```python
from build123d import *

# Parameters (mm, degrees)
SKETCH1_W           = 250
SKETCH1_H           = 100
SKETCH1_R           = 5
SKETCH1_R_2         = 2.5
BOSS_EXTRUDE1_DEPTH = 5
BOSS_EXTRUDE2_DEPTH = 10
CUT_EXTRUDE1_DEPTH  = 5
SKETCH4_R           = 4
CUT_EXTRUDE2_DEPTH  = 44.5
SKETCH5_W           = 5
SKETCH5_H           = 5
SKETCH5_W_2         = 2.5
CUT_EXTRUDE3_DEPTH  = 290.5
SKETCH6_W           = 5
SKETCH6_H           = 5
CUT_EXTRUDE4_DEPTH  = 290.5


with BuildPart() as part:
    # Sketch1 → Boss-Extrude1 (new, symmetric)
    with BuildSketch(Plane(origin=(0, 0, 0), x_dir=(1, 0, 0), z_dir=(0, 1, 0))):
        Rectangle(SKETCH1_W, SKETCH1_H)
        with Locations(Location((-100, 40, 0), (0, 0, 270))):
            Circle(SKETCH1_R, mode=Mode.SUBTRACT)
        with Locations(Location((100, 40, 0), (0, 0, 270))):
            Circle(SKETCH1_R, mode=Mode.SUBTRACT)
        with Locations(Location((-100, -40, 0), (0, 0, 90))):
            Circle(SKETCH1_R, mode=Mode.SUBTRACT)
        with Locations(Location((100, -40, 0), (0, 0, 90))):
            Circle(SKETCH1_R, mode=Mode.SUBTRACT)
        with Locations(Location((-20, 20, 0), (0, 0, 270))):
            Circle(SKETCH1_R_2, mode=Mode.SUBTRACT)
        with Locations(Location((20, 20, 0), (0, 0, 270))):
            Circle(SKETCH1_R_2, mode=Mode.SUBTRACT)
        with Locations(Location((-20, -20, 0), (0, 0, 270))):
            Circle(SKETCH1_R_2, mode=Mode.SUBTRACT)
        with Locations(Location((20, -20, 0), (0, 0, 270))):
            Circle(SKETCH1_R_2, mode=Mode.SUBTRACT)
        with Locations(Location((-115, 0, 0), (0, 0, 270))):
            Circle(SKETCH1_R_2, mode=Mode.SUBTRACT)
        with Locations(Location((-105, 0, 0), (0, 0, 270))):
            Circle(SKETCH1_R_2, mode=Mode.SUBTRACT)
        with Locations(Location((-95, 0, 0), (0, 0, 270))):
            Circle(SKETCH1_R_2, mode=Mode.SUBTRACT)
        with Locations(Location((-85, 0, 0), (0, 0, 270))):
            Circle(SKETCH1_R_2, mode=Mode.SUBTRACT)
        with Locations(Location((-75, 0, 0), (0, 0, 270))):
            Circle(SKETCH1_R_2, mode=Mode.SUBTRACT)
        with Locations(Location((75, 0, 0), (0, 0, 90))):
            Circle(SKETCH1_R_2, mode=Mode.SUBTRACT)
        with Locations(Location((85, 0, 0), (0, 0, 90))):
            Circle(SKETCH1_R_2, mode=Mode.SUBTRACT)
        with Locations(Location((95, 0, 0), (0, 0, 90))):
            Circle(SKETCH1_R_2, mode=Mode.SUBTRACT)
        with Locations(Location((105, 0, 0), (0, 0, 90))):
            Circle(SKETCH1_R_2, mode=Mode.SUBTRACT)
        with Locations(Location((115, 0, 0), (0, 0, 90))):
            Circle(SKETCH1_R_2, mode=Mode.SUBTRACT)
    extrude(amount=BOSS_EXTRUDE1_DEPTH, both=True)

    # Sketch2 → Boss-Extrude2 (add, symmetric)
    with BuildSketch(Plane(origin=(0, 0, 0), x_dir=(0, 0, -1), z_dir=(1, 0, 0))):
        with BuildLine():
            Line((55, -5), (50, -5))
            Line((50, -5), (50, 0))
            ThreePointArc((50, 0), (58.535533906, 3.535533906), (55, -5))
        make_face()
    extrude(amount=BOSS_EXTRUDE2_DEPTH, both=True)

    # Sketch3 → Cut-Extrude1 (cut, symmetric)
    with BuildSketch(Plane(origin=(0, 0, 0), x_dir=(0, 0, -1), z_dir=(1, 0, 0))):
        Polygon((50, 5), (50, -6.022521845), (64.637798631, -7.270431104), (61.921760831, 9.282718187), align=None)
    extrude(amount=CUT_EXTRUDE1_DEPTH, both=True, mode=Mode.SUBTRACT)

    # Sketch4 → Cut-Extrude2 (cut, symmetric)
    with BuildSketch(Plane(origin=(10, 0, 0), x_dir=(0, 0, -1), z_dir=(1, 0, 0))):
        with Locations((55, 0)):
            Circle(SKETCH4_R)
    extrude(amount=CUT_EXTRUDE2_DEPTH, both=True, mode=Mode.SUBTRACT)

    # Sketch5 → Cut-Extrude3 (cut, symmetric)
    with BuildSketch(Plane(origin=(125, 0, 0), x_dir=(0, 0, -1), z_dir=(1, 0, 0))):
        with Locations((-50, 5)):
            Rectangle(SKETCH5_W, SKETCH5_H)
        with Locations((48.75, 5)):
            Rectangle(SKETCH5_W_2, SKETCH5_H)
    extrude(amount=CUT_EXTRUDE3_DEPTH, both=True, mode=Mode.SUBTRACT)

    # Sketch6 → Cut-Extrude4 (cut, symmetric)
    with BuildSketch(Plane.XY):
        with Locations((125, 5)):
            Rectangle(SKETCH6_W, SKETCH6_H)
        with Locations((-125, 5)):
            Rectangle(SKETCH6_W, SKETCH6_H)
    extrude(amount=CUT_EXTRUDE4_DEPTH, both=True, mode=Mode.SUBTRACT)


solid = part.part
```
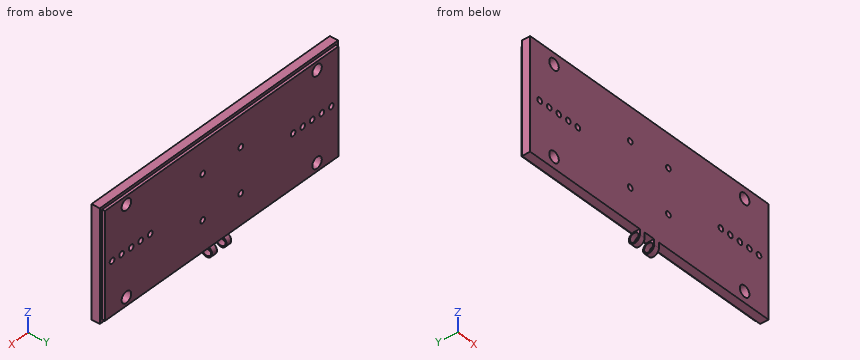
Source: CAD feature listing. Evaluate the final solid. Frame: model axes, mm. Round coordinates to 2 decimals unless told otherwise and drop trailing zeros. Loops run counter-clockwise (first coordinate to the right, second up) from the corner with the lowest first, then second, coordinate; pieces in that order, holes last.
(1) Section query C-C (x = 44.5). Output: boundary loops of the cut face in (y, z).
From the geometry:
outline: (-5, -50) - (2.5, -50) - (2.5, -47.5) - (5, -47.5) - (5, 47.5) - (2.5, 47.5) - (2.5, 50) - (-5, 50) - close
(2) Section query A-A (x = -75). Output: boundary loops of the cut face in (y, z), and give its area (4 significant figures).
From the geometry:
outline: (-5, -50) - (2.5, -50) - (2.5, -47.5) - (5, -47.5) - (5, -2.5) - (-5, -2.5) - close; (-5, 2.5) - (5, 2.5) - (5, 47.5) - (2.5, 47.5) - (2.5, 50) - (-5, 50) - close
area: 937.5 mm2
(3) Section query D-D (y = -2). Give the number of separate pieces and of enclosed holes in the cut face, and give its area (3 significant figures).
From the geometry:
separate pieces: 3
enclosed holes: 18
area: 24,400 mm2
(4) Contact query for flat-ended pins moving along their axis: pin 1 Ø2 at (x, y) = (21.5, -1.5) entering from -Z; pin 2 Ø1 at (y, z) = (3.5, 18) entering from +X; pin 3 Ø1.2 at (x, y) = (18, 3.5) entering from +Z. Output: stop coordinate, or through.
From the geometry:
pin 1: stops at z = -50
pin 2: stops at x = 122.5
pin 3: stops at z = 47.5
(5) Material intervals for probe 1 along X at (y, z) = (0, 40); probe 2 along X at (y, z) = (4.5, -40); probe 3 along Z at (x, y) = (-2, 4), sorted ascending.
From the geometry:
probe 1: x = -125 to -105, -95 to 95, 105 to 125
probe 2: x = -122.5 to -105, -95 to 95, 105 to 122.5
probe 3: z = -47.5 to 47.5
(6) Section query B-B (z = 20). Output: boundary loops of the cut face in (x, y), and give its area (3 significant figures).
From the geometry:
outline: (-125, -5) - (-22.5, -5) - (-22.5, 5) - (-122.5, 5) - (-122.5, 2.5) - (-125, 2.5) - close; (-17.5, -5) - (17.5, -5) - (17.5, 5) - (-17.5, 5) - close; (22.5, -5) - (125, -5) - (125, 2.5) - (122.5, 2.5) - (122.5, 5) - (22.5, 5) - close
area: 2,390 mm2
